```python
from build123d import *

# Parameters (mm, degrees)
F0_R            = 1.75
F0_R_2          = 11
F1_DEPTH        = 6
F2_SIZE         = 1
F4_DEPTH        = 24
F5_DEPTH        = 10
F6_SIZE         = 1
F8_D            = 4.4
F8_CBORE_D      = 8.25
F8_CBORE_DEPTH  = 4
F10_D           = 4.4
F10_CBORE_D     = 8.25
F10_CBORE_DEPTH = 4
F11_W           = 6
F11_H           = 24
F12_DEPTH       = 25
F13_W           = 5
F13_H           = 24
F14_DEPTH       = 43
F15_SIZE        = 24
F16_R           = 5


with BuildPart() as f1:
    # F0 (on Top) → F1 (new body)
    with BuildSketch(Plane.XY):
        Polygon((18.8770524859, 25.5778683759), (-30.1229475141, 25.5778683759), (-30.1229475141, -25.4221316241), (18.8770524859, -25.4221316241), (18.8770524859, -5.4221316241), align=None)
        with Locations((-24.6229475141, -10.9221316241)):
            Circle(F0_R, mode=Mode.SUBTRACT)
        with Locations((6.3770524859, -10.9221316241)):
            Circle(F0_R, mode=Mode.SUBTRACT)
        with Locations((-9.1229475141, 4.5778683759)):
            Circle(F0_R_2, mode=Mode.SUBTRACT)
        with Locations((-24.6229475141, 20.0778683759)):
            Circle(F0_R, mode=Mode.SUBTRACT)
        with Locations((6.3770524859, 20.0778683759)):
            Circle(F0_R, mode=Mode.SUBTRACT)
        Polygon((22.8770524859, 25.5778683759), (18.8770524859, 25.5778683759), (18.8770524859, -5.4221316241), (38.8770524859, -5.4221316241), (38.8770524859, 14.5778683759), (30.8770524859, 14.5778683759), align=None)
    extrude(amount=F1_DEPTH)

    # F2
    f2_edges = [f1.edges().sort_by_distance(p)[0] for p in [
        (-26.372948, 20.077868, 0),
        (4.627052, 20.077868, 0),
        (4.627052, -10.922132, 0),
        (-26.372948, -10.922132, 0),
    ]]
    chamfer(f2_edges, length=F2_SIZE)

    # F3 (on face) → F4 (join)
    with BuildSketch(Plane.XY.offset(6)):
        Polygon((18.8770524859, -25.4221316241), (18.8770524859, -5.4221316241), (38.8770524859, -5.4221316241), (38.8770524859, 0.5778683759), (12.8770524859, 0.5778683759), (12.8770524859, -25.4221316241), align=None)
    extrude(amount=F4_DEPTH)

    # F3 (on face) → F5 (join)
    with BuildSketch(Plane.XY.offset(6)):
        Polygon((18.8770524859, -25.4221316241), (18.8770524859, -5.4221316241), (38.8770524859, -5.4221316241), (38.8770524859, 0.5778683759), (12.8770524859, 0.5778683759), (12.8770524859, -25.4221316241), align=None)
    extrude(amount=F5_DEPTH)

    # F6
    f6_edges = [f1.edges().sort_by_distance(p)[0] for p in [
        (18.877052, -5.422132, 15),
    ]]
    chamfer(f6_edges, length=F6_SIZE)

    # F8 (through all)
    with Locations(Plane(origin=(0, 0.5778683759, 0), x_dir=(-1, 0, 0), z_dir=(0, 1, 0))):
        with Locations((-28.8770524859, 25), (-28.8770524859, 11)):
            CounterBoreHole(F8_D / 2, F8_CBORE_D / 2, F8_CBORE_DEPTH)

    # F10 (through all)
    with Locations(Plane(origin=(12.8770524859, 0, 0), x_dir=(0, -1, 0), z_dir=(-1, 0, 0))):
        with Locations((15.4221316241, 25), (15.4221316241, 11)):
            CounterBoreHole(F10_D / 2, F10_CBORE_D / 2, F10_CBORE_DEPTH)

    # F11 (on face) → F12 (join, through all)
    with BuildSketch(Plane(origin=(0, 0.5778683759, 0), x_dir=(-1, 0, 0), z_dir=(0, 1, 0))):
        with Locations((-15.8770524859, 18)):
            Rectangle(F11_W, F11_H)
    extrude(amount=F12_DEPTH)

    # F13 (on face) → F14 (join, through all)
    with BuildSketch(Plane(origin=(12.8770524859, 0, 0), x_dir=(0, -1, 0), z_dir=(-1, 0, 0))):
        with Locations((22.9221316241, 18)):
            Rectangle(F13_W, F13_H)
    extrude(amount=F14_DEPTH)

    # F15
    f15_edges = [f1.edges().sort_by_distance(p)[0] for p in [
        (-30.122948, -22.922132, 30),
        (15.877052, 25.577868, 30),
    ]]
    chamfer(f15_edges, length=F15_SIZE)

    # F16
    f16_edges = [f1.edges().sort_by_distance(p)[0] for p in [
        (30.877052, 14.577868, 3),
        (22.877052, 25.577868, 3),
        (38.877052, 14.577868, 3),
        (-30.122948, -25.422132, 3),
        (-30.122948, 25.577868, 3),
    ]]
    fillet(f16_edges, radius=F16_R)


solid = f1.part
```
Input: part model. Units: mm. Frame: model coordinates. A direction names the side the tool comes from. Coordinates: 2 decimals unless noted, no trailing zeros. Order: outer loops, then holes, each group sorted by start corner. A loop starts at its lowest first (then second) coordinate and runs counter-clockwise, first axis right, second up. Notation, with made-up numbers: (-32.75, -15.5) - (14.25, -15.5) arc R21 cw to (14.25, -10.5) - close; hole circle Ø8 at (34, -16.75). An arc over 180 degrees is marked (long way). Put each result on its own line as item: value.
1. Contact query for flat-ended pins moving along their axis: pin 1 Ø4 at (x, z) = (30.5, 9) entering from +Y; pin 2 Ø6.5 at (y, z) = (-15.42, 25) entering from -X; pin 3 Ø3 at (y, z) = (14, 15.5) entering from -X. Output: stop coordinate, or through.
Report:
pin 1: stops at y = 0.58
pin 2: stops at x = 16.88
pin 3: stops at x = 12.88
2. Cut plane A-A on z = 10. Return the cut outline in (x, y), then the cut area to 3 significant figures.
Report:
outline: (-26.12, -25.32) arc R5 ccw to (-25.12, -25.42) - (18.88, -25.42) - (18.88, -17.38) - (16.88, -17.38) - (16.88, -19.42) - (12.88, -19.42) - (12.88, -20.42) - (-26.12, -20.42) - close; (12.88, -11.42) - (16.88, -11.42) - (16.88, -13.46) - (18.88, -13.46) - (18.88, -6.42) - (19.88, -5.42) - (26.92, -5.42) - (26.92, -3.42) - (24.88, -3.42) - (24.88, 0.58) - (18.88, 0.58) - (18.88, 21.58) - (12.88, 21.58) - close; (30.84, -5.42) - (38.88, -5.42) - (38.88, 0.58) - (32.88, 0.58) - (32.88, -3.42) - (30.84, -3.42) - close
area: 518 mm2
3. Draft query along X for faces 5 (the face through (-3, -25.422, 15)), 6 (the face through (16.877, -17, 23)), 7 (the face through (-25.913, 21.261, 3.465)). Return one class per face: pulls with the +X half, pulls with the -X half, needs draft (parallel to the pull), parting line crosses it, or undercut.
Report:
face 5: needs draft
face 6: pulls with the -X half
face 7: undercut
4. Cut plane D-D on z = 25. Return the cut outline in (x, y), then the cut area to 3 significant figures.
Report:
outline: (-11.12, -25.42) - (18.88, -25.42) - (18.88, -17.62) - (16.88, -17.62) - (16.88, -19.55) - (12.88, -19.55) - (12.88, -20.42) - (-11.12, -20.42) - close; (12.88, -11.3) - (16.88, -11.3) - (16.88, -13.22) - (18.88, -13.22) - (18.88, -6.42) - (19.88, -5.42) - (26.68, -5.42) - (26.68, -3.42) - (24.75, -3.42) - (24.75, 0.58) - (18.88, 0.58) - (18.88, 6.58) - (12.88, 6.58) - close; (31.08, -5.42) - (38.88, -5.42) - (38.88, 0.58) - (33, 0.58) - (33, -3.42) - (31.08, -3.42) - close
area: 349 mm2
5. Reachability of faces 1 (the face through (14.849, -14.528, 6.973)), 2 (the face through (26.66, -1.39, 28.48)), 3 (the face through (18.877, -16, 15)), 4 (the face through (12.877, -3, 15)) from +Z, -Z, +X, -X, +Y, -Y: full face, straight path, thin tool, end or side. Return the list, or none.
Report:
face 1: -X
face 2: +Y
face 3: +Z, -Z, +X, -Y
face 4: +Z, -X, +Y
6. Line query: line 1 along Z through (x, y) = (16.5, -16); line 2 along Y through (x, z) = (8, 13.5); line 3 along Z through (x, y) = (-14.5, 19). Output: solid intervals per line, ascending.
Report:
line 1: z = 0 to 6.92, 15.08 to 20.92, 29.08 to 30
line 2: y = -25.42 to -20.42
line 3: z = 0 to 6
7. Cut plane C-C on z = 18. Return the cut outline in (x, y).
Report:
outline: (-18.12, -25.42) - (18.88, -25.42) - (18.88, -6.42) - (19.88, -5.42) - (38.88, -5.42) - (38.88, 0.58) - (18.88, 0.58) - (18.88, 13.58) - (12.88, 13.58) - (12.88, -20.42) - (-18.12, -20.42) - close
8. Cut plane B-B on x = -1. Return the cut outline in (y, z), then the cut area to 3 significant figures.
Report:
outline: (-25.42, 0) - (-2.84, 0) - (-2.84, 6) - (-20.42, 6) - (-20.42, 30) - (-25.42, 30) - close; (12, 0) - (25.58, 0) - (25.58, 6) - (12, 6) - close
area: 337 mm2
